Source: CAD feature listing. Evaluate the final solid. Frame: model axes, mm. Face numbers are marked on the shaded views. A direction names the side the tool comes from. Give positions to 0.01 mm unless a question says otherwise; leave off trailing zeros. Loops run counter-clockwise (first coordinate to the right, second up) from the corner with the lowest first, then second, coordinate; pieces in that order, holes last. Notation, with made-up numbers: M -32,36.25 L 3,36.25 A22 cw 3,72.25 Z; hole C -5,87.25 d2. An arc over 180 degrees is marked long. Write item = value, one per line.
from build123d import *

# Parameters (mm, degrees)
SKETCH1_R           = 3.75
BOSS_EXTRUDE1_DEPTH = 8
SKETCH2_R           = 3.75
SKETCH2_R_2         = 2.5
CUT_EXTRUDE1_DEPTH  = 4
SKETCH3_R           = 1.65
BOSS_EXTRUDE2_DEPTH = 2


with BuildPart() as part:
    # Sketch1 → Boss-Extrude1 (new body)
    with BuildSketch(Plane(origin=(0, 0, 0), x_dir=(1, 0, 0), z_dir=(0, 1, 0))):
        Circle(SKETCH1_R)
    extrude(amount=BOSS_EXTRUDE1_DEPTH)

    # Sketch2 → Cut-Extrude1 (cut)
    with BuildSketch(Plane(origin=(0, 8, 0), x_dir=(1, 0, 0), z_dir=(0, 1, 0))):
        Circle(SKETCH2_R)
        Circle(SKETCH2_R_2, mode=Mode.SUBTRACT)
    extrude(amount=-CUT_EXTRUDE1_DEPTH, mode=Mode.SUBTRACT)

    # Sketch3 → Boss-Extrude2 (add)
    with BuildSketch(Plane(origin=(0, 8, 0), x_dir=(1, 0, 0), z_dir=(0, 1, 0))):
        Circle(SKETCH3_R)
    extrude(amount=BOSS_EXTRUDE2_DEPTH)


solid = part.part
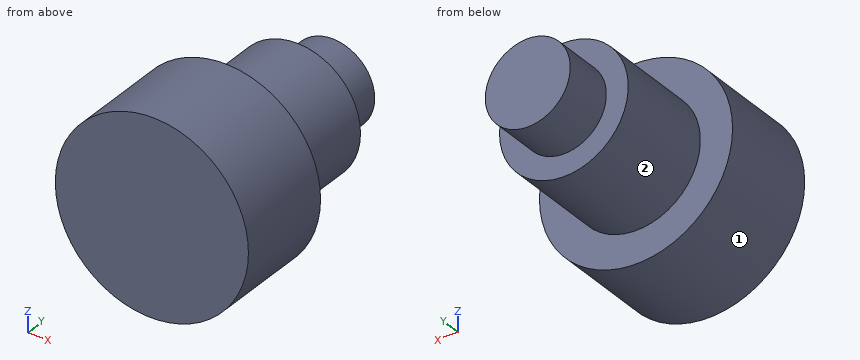
1. Cut plane B-B, the plane x = 0. Return the cut outline in (y, z), then the cut area to 3 significant figures.
Derived:
outline = M 0,-3.75 L 4,-3.75 L 4,-2.5 L 8,-2.5 L 8,-1.65 L 10,-1.65 L 10,1.65 L 8,1.65 L 8,2.5 L 4,2.5 L 4,3.75 L 0,3.75 Z
area = 56.6 mm²
2. First-contact query: pin 1 Ø1 at (y, z) = (6, -1.5) entering from -X. Flat tip, straight axial feed; report the tip coordinate or a pass-through.
Derived:
pin_1 = -2.29
3. Cut plane A-A, the plane z = 0. Return the cut outline in (x, y).
Derived:
outline = M -3.75,0 L 3.75,0 L 3.75,4 L 2.5,4 L 2.5,8 L 1.65,8 L 1.65,10 L -1.65,10 L -1.65,8 L -2.5,8 L -2.5,4 L -3.75,4 Z
4. Material intervals for probe 1 along Y at (x, z) = (-0.5, -3); probe 2 along Y at (x, z) = (-0.75, 2); probe 3 along Z at (x, y) = (-1.25, 1.5), sorted ascending. Write a range as from..to.
Derived:
probe_1 = 0..4
probe_2 = 0..8
probe_3 = -3.54..3.54
5. Reachability of the marked faces 1 and 2 from +Z, -Z, +X, -X, +Y, -Y: full face, straight path, thin tool, end or side. Return the list, or none.
Derived:
face_1 = +Y, -Y
face_2 = +Y
6. Cut plane C-C, the plane y = 5. Return the cut outline in (x, z), then the cut area to 3 significant figures.
Derived:
outline = C 0,0 d5
area = 19.6 mm²
7. Cut plane D-D, the plane x = -2. Return the cut outline in (y, z), then the cut area to 3 significant figures.
Derived:
outline = M 0,-3.17 L 4,-3.17 L 4,-1.5 L 8,-1.5 L 8,1.5 L 4,1.5 L 4,3.17 L 0,3.17 Z
area = 37.4 mm²
